Here's the drawing with two shaded views (mm, measured from the low corner). I have some questions. Coordinates: 2 decimals unless noted, no trailing zeros. Loops run counter-clockwise (first coordinate to the right, second up) from the corner with the lowest first, then second, coordinate; pieces in that order, holes last. Notation, with made-up numbers: (24, 67.5) -> (59, 67.5) arc R21 ccw to (59, 99.5) -> close; hole circle Ø11 at (-35.75, 41). An arc over 180 degrees is marked (long way). Answer as a JSON object with one key per item and string values. Group by question number.
1) I need wall thicknesses on probe 1 along Z at (x, y) = (88.5, 5.25); probe 2 along X at (y, z) = (1, 28.5); probe 3 along Z at (x, y) = (147, 1.5). Which ranges of each line are inside material? Lowest first, please. Write a range as [from, to].
2) I want a section at A-A (z = 19). Write out the boundary of the cut face in (x, y).
3) I want a section at D-D (z = 34.5). Write out the boundary of the cut face in (x, y).
4) If we mould it in two halves opening along X, with no side actions, what happens to the marked faces 1, 2 and 3? For each: +X half, -X half, draft (parallel to the pull), parting line (faces both ways), or undercut.
5) I want a section at B-B (x = 147). Write out the boundary of the cut face in (y, z).
6) I want a section at C-C (y = 1.75). Write out the boundary of the cut face in (x, z), then the cut area to 3 significant figures.
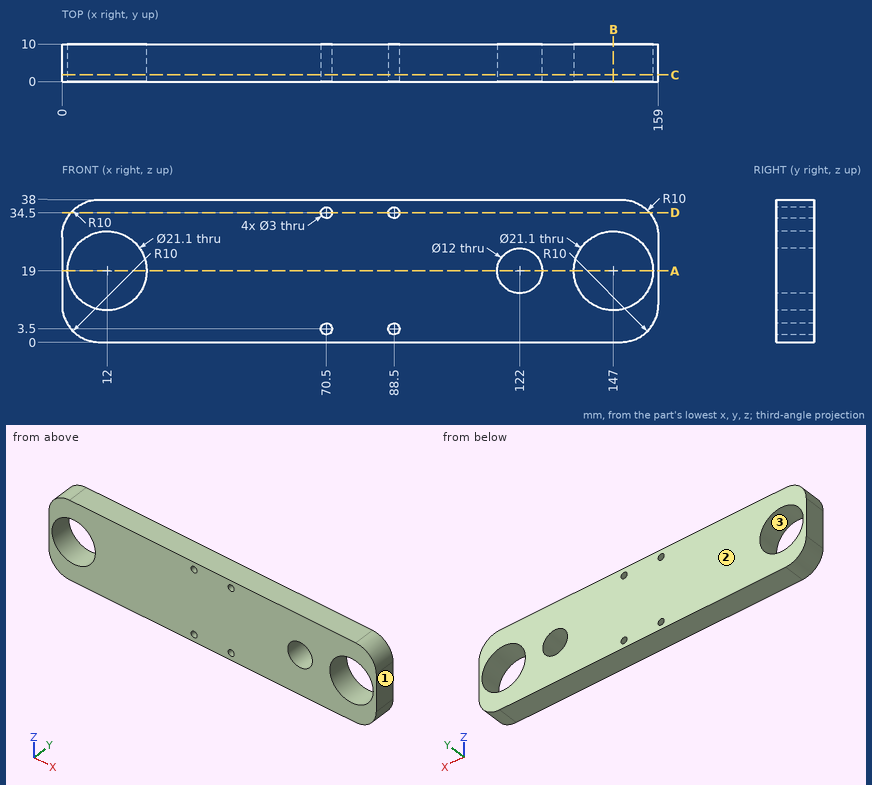
Determined:
{
 "1": {"probe 1": "[0, 2], [5, 33], [36, 38]", "probe 2": "[0.01, 7.41], [16.59, 142.41], [151.59, 158.99]", "probe 3": "[0, 8.45], [29.55, 38]"},
 "2": {"outline": "(0, 0) -> (1.45, 0) -> (1.45, 10) -> (0, 10) -> close; (22.55, 0) -> (116, 0) -> (116, 10) -> (22.55, 10) -> close; (128, 0) -> (136.45, 0) -> (136.45, 10) -> (128, 10) -> close; (157.55, 0) -> (159, 0) -> (159, 10) -> (157.55, 10) -> close"},
 "3": {"outline": "(2.4, 0) -> (69, 0) -> (69, 10) -> (2.4, 10) -> close; (72, 0) -> (87, 0) -> (87, 10) -> (72, 10) -> close; (90, 0) -> (156.6, 0) -> (156.6, 10) -> (90, 10) -> close"},
 "4": {"face 1": "+X half", "face 2": "draft", "face 3": "undercut"},
 "5": {"outline": "(0, 0) -> (10, 0) -> (10, 8.45) -> (0, 8.45) -> close; (0, 29.55) -> (10, 29.55) -> (10, 38) -> (0, 38) -> close"},
 "6": {"outline": "(0, 10) arc R10 ccw to (10, 0) -> (149, 0) arc R10 ccw to (159, 10) -> (159, 28) arc R10 ccw to (149, 38) -> (10, 38) arc R10 ccw to (0, 28) -> close; hole circle Ø21.1 at (12, 19); hole circle Ø3 at (70.5, 3.5); hole circle Ø3 at (70.5, 34.5); hole circle Ø3 at (88.5, 3.5); hole circle Ø3 at (88.5, 34.5); hole circle Ø12 at (122, 19); hole circle Ø21.1 at (147, 19)", "area": "5,120 mm^2"}
}
